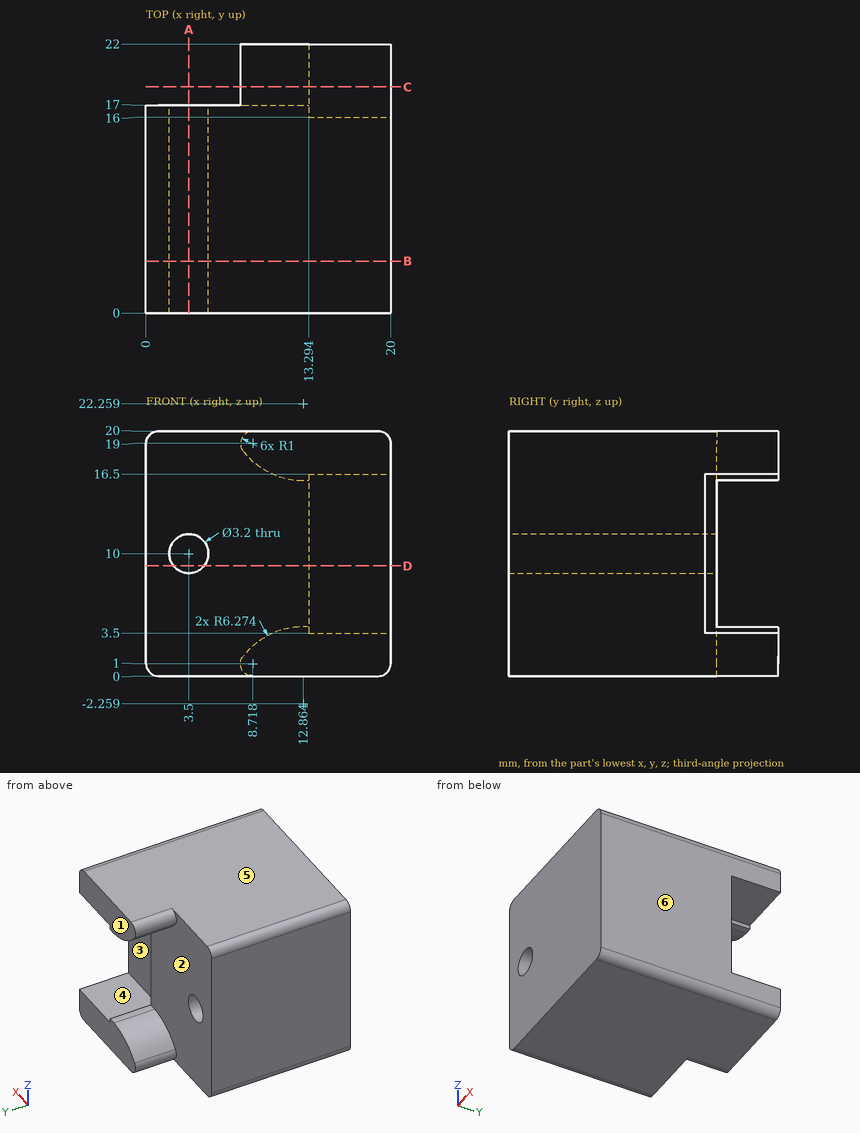
Check sheet for the drawn part. Datum: minimum x, y, z corner. Units: mm. A direction names the side the tool comes from. Give positions to 0.01 mm unless a question says otherwise; leave off trailing zeros. Order: outer loops, then holes, each group sorted by start corner. A loop starts at its lowest first (then second) coordinate and runs counter-clockwise, first axis right, second up. Notation, with made-up numbers: (22, 58) - (48, 58) arc R13 cw to (48, 73) - close; hole circle Ø8 at (-8.5, -17). An arc over 180 degrees is marked (long way). Answer as a JSON object with one key per item and string values.
(1) Cross-section at B-B (y = 4.25). Record the cut outline in (x, z).
Report:
{"outline": "(0, 1) arc R1 ccw to (1, 0) - (19, 0) arc R1 ccw to (20, 1) - (20, 19) arc R1 ccw to (19, 20) - (1, 20) arc R1 ccw to (0, 19) - close; hole circle Ø3.2 at (3.5, 10)"}
(2) Cross-section at C-C (y = 18.5). Record the cut outline in (x, z) (1 decimal).
Report:
{"outline": "(7.9, 1.6) arc R1 ccw to (8.7, 0) - (19, 0) arc R1 ccw to (20, 1) - (20, 3.5) - (13.3, 3.5) - (13.3, 4) arc R6.3 ccw to start; (7.9, 18.4) arc R6.3 ccw to (13.3, 16) - (13.3, 16.5) - (20, 16.5) - (20, 19) arc R1 ccw to (19, 20) - (8.7, 20) arc R1 ccw to start"}
(3) Draft check along Z on the marked faces 4, 5 and 6. Enter one of: released by +Z, released by -Z, zero draft, split by the parting line, or undercut.
Report:
{"face 4": "undercut", "face 5": "released by +Z", "face 6": "zero draft"}
(4) Tool access check on the marked faces 1, 2 and 3. Record the directions out of +Z, -Z, +X, -X, +Y, -Y that give a thin tool (end or side, any length) a straight path to the whole face; none if there is none.
Report:
{"face 1": "+Z, -Z, +X, -X, +Y", "face 2": "-X, +Y", "face 3": "+X, +Y"}
(5) Cross-section at A-A (x = 3.5). Record the cut outline in (y, z), then the cut area to 3 significant figures.
Report:
{"outline": "(0, 0) - (17, 0) - (17, 8.4) - (0, 8.4) - close; (0, 11.6) - (17, 11.6) - (17, 20) - (0, 20) - close", "area": "286 mm^2"}
(6) Depth check by flat-ended pin: pin 1 Ø4 at (x, z) = (3.5, 10) entering from +Y; pin 2 Ø7.5 at (x, z) = (18, 12) entering from +Y. Enter the tip coordinate at first touch or a pass-through.
Report:
{"pin 1": "y = 17", "pin 2": "y = 16"}
(7) Cross-section at D-D (z = 9). Record the cut outline in (x, y) (1 decimal), then the cut area to 3 significant figures.
Report:
{"outline": "(0, 0) - (2.3, 0) - (2.3, 17) - (0, 17) - close; (4.7, 0) - (20, 0) - (20, 16) - (13.3, 16) - (13.3, 17) - (4.7, 17) - close", "area": "291 mm^2"}
(8) Material ranges on line 1 (Z direction, x = 3.5, y = 3.25); line 2 (X direction, y = 16.3, z = 10) (1 decimal); line 3 (Y direction, x = 7.5, z = 5.75), recorded low to high.
Report:
{"line 1": "0 to 8.4, 11.6 to 20", "line 2": "0 to 1.9, 5.1 to 13.3", "line 3": "0 to 17"}
